Check sheet for the modelled part. Datum: model origin and axes. Units: mm. Face numbers are marked on the shaded views. A direction names the side the tool comes from. Coordinates: 2 decimals unless noted, no trailing zeros. Write each loop counter-clockwise with the first axis right and the second up, starting at its lowest first coordinate (ties: lowest second). Pieces come first, ordered by that corner, then holes. Notation, with made-up numbers: M 5.25,77.5 L 62.25,77.5 A21 ccw 62.25,86.5 Z; hole C 6.25,41.25 d6. An arc over 180 degrees is marked long. Answer as CSV lines item,"result". Start each with the question number.
Q1. Depth check by flat-ended pin: pin 1 Ø1.2 at (x, z) = (-8, -10) entering from +Y; pin 2 Ø1.5 at (x, y) = (-11.5, -3) entering from +Z; pin 3 Ø1.3 at (x, y) = (-26, -6.5) entering from -Z. Enter the tip coordinate at first touch or a pass-through.
Q2. Sectioned sample at D-D, the plane y = -2.5. Count the separate pieces of the cut face and the enclosed holes in it, then the cut area to 3 significant figures.
Q3. Sectioned sample at B-B, the plane x = 0. Record the cut outline in (y, z).
Q4. Sectioned sample at A-A, the plane z = 0. Record the cut outline in (x, y), then the cut area to 3 significant figures.
Q5. Mould release check, pull along X, two halves, no side actions. Record for the marked faces 3, 4 and 5: pulls with the +X half, pulls with the -X half, needs draft (parallel to the pull), parting line crosses it, or undercut.
Q6. Access from +Z, -Z, +X, -X, +Y, -Y to the whole of each face (thin tool, end or side, straight path). Record for the marked faces 1 and 2.
Q7. Thickness scan on line 1 along X through (y, z) = (-2, -26); line 2 along X through (y, z) = (-2.5, 26.25); line 3 along X through (y, z) = (-5.9, 0). Record the ranges inside material, lowest first. Write a range as from..to.
Q8. Sectioned sample at C-C, the plane z = -26.25. Record the cut outline in (x, y).
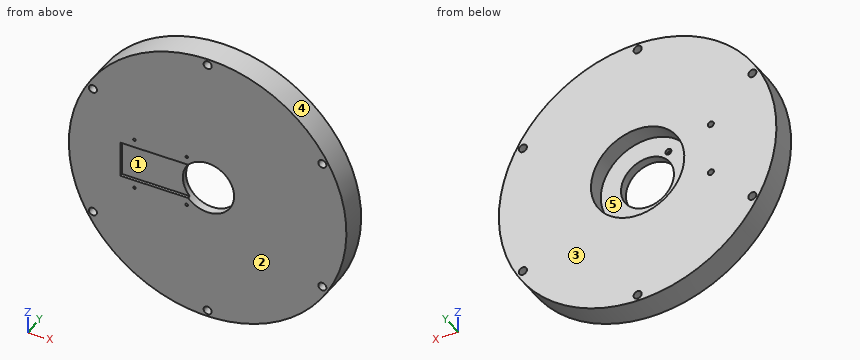
from build123d import *

# Parameters (mm, degrees)
SKETCH1_R           = 55
SKETCH1_R_2         = 50
SKETCH1_R_3         = 1.6
BOSS_EXTRUDE1_DEPTH = 7.5
SKETCH2_3_R         = 50
SKETCH2_3_R_2       = 10.5
BOSS_EXTRUDE2_DEPTH = 7.5
SKETCH2_R           = 0.5
CUT_EXTRUDE1_DEPTH  = 7.5
SKETCH2_3_2_R       = 1.2
SKETCH2_3_2_R_2     = 0.5
CUT_EXTRUDE2_DEPTH  = 5.3
CUT_EXTRUDE3_START  = -1.2
CUT_EXTRUDE3_DEPTH  = 1.2
SKETCH4_R           = 18.5
CUT_EXTRUDE4_DEPTH  = 4
BOSS_EXTRUDE3_START = 3
SKETCH5_R           = 55
SKETCH5_R_2         = 18.5
SKETCH5_R_3         = 1.6
SKETCH5_R_4         = 1.2
BOSS_EXTRUDE3_DEPTH = 3


with BuildPart() as part:
    # Sketch1 → Boss-Extrude1 (new body)
    with BuildSketch(Plane(origin=(0, 0, 0), x_dir=(1, 0, 0), z_dir=(0, 1, 0))):
        with Locations(Location((0, 0, 0), (0, 0, 270))):
            Circle(SKETCH1_R)
        with Locations(Location((0, 0, 0), (0, 0, 270))):
            Circle(SKETCH1_R_2, mode=Mode.SUBTRACT)
        with Locations(Location((0, 52.5, 0), (0, 0, 270))):
            Circle(SKETCH1_R_3, mode=Mode.SUBTRACT)
        with Locations(Location((45.466333699, 26.25, 0), (0, 0, 270))):
            Circle(SKETCH1_R_3, mode=Mode.SUBTRACT)
        with Locations(Location((45.466333699, -26.25, 0), (0, 0, 270))):
            Circle(SKETCH1_R_3, mode=Mode.SUBTRACT)
        with Locations(Location((0, -52.5, 0), (0, 0, 270))):
            Circle(SKETCH1_R_3, mode=Mode.SUBTRACT)
        with Locations(Location((-45.466333699, -26.25, 0), (0, 0, 270))):
            Circle(SKETCH1_R_3, mode=Mode.SUBTRACT)
        with Locations(Location((-45.466333699, 26.25, 0), (0, 0, 270))):
            Circle(SKETCH1_R_3, mode=Mode.SUBTRACT)
    extrude(amount=-BOSS_EXTRUDE1_DEPTH)

    # Sketch2_3 → Boss-Extrude2 (add)
    with BuildSketch(Plane(origin=(0, 0, 0), x_dir=(1, 0, 0), z_dir=(0, 1, 0))):
        Circle(SKETCH2_3_R)
        with Locations(Location((0, 0, 0), (0, 0, 270))):
            Circle(SKETCH2_3_R_2, mode=Mode.SUBTRACT)
    extrude(amount=-BOSS_EXTRUDE2_DEPTH)

    # Sketch2 → Cut-Extrude1 (cut)
    with BuildSketch(Plane(origin=(0, 0, 0), x_dir=(1, 0, 0), z_dir=(0, 1, 0))):
        with Locations(Location((-29, 10.25, 0), (0, 0, 270))):
            Circle(SKETCH2_R)
        with Locations(Location((-8.3, 10.25, 0), (0, 0, 270))):
            Circle(SKETCH2_R)
        with Locations(Location((-8.3, -10.25, 0), (0, 0, 270))):
            Circle(SKETCH2_R)
        with Locations(Location((-29, -10.25, 0), (0, 0, 270))):
            Circle(SKETCH2_R)
    extrude(amount=-CUT_EXTRUDE1_DEPTH, mode=Mode.SUBTRACT)

    # Sketch2_3 2 → Cut-Extrude2 (cut)
    # profile 1 of 4: a face of its own
    with BuildSketch(Plane(origin=(0, 0, 0), x_dir=(1, 0, 0), z_dir=(0, 1, 0))):
        with Locations(Location((-29, 10.25, 0), (0, 0, 270))):
            Circle(SKETCH2_3_2_R)
        with Locations(Location((-29, 10.25, 0), (0, 0, 270))):
            Circle(SKETCH2_3_2_R_2, mode=Mode.SUBTRACT)
    # profile 2 of 4: a face of its own
    with BuildSketch(Plane(origin=(0, 0, 0), x_dir=(1, 0, 0), z_dir=(0, 1, 0))):
        with Locations(Location((-8.3, 10.25, 0), (0, 0, 270))):
            Circle(SKETCH2_3_2_R)
        with Locations(Location((-8.3, 10.25, 0), (0, 0, 270))):
            Circle(SKETCH2_3_2_R_2, mode=Mode.SUBTRACT)
    # profile 3 of 4: a face of its own
    with BuildSketch(Plane(origin=(0, 0, 0), x_dir=(1, 0, 0), z_dir=(0, 1, 0))):
        with Locations(Location((-8.3, -10.25, 0), (0, 0, 270))):
            Circle(SKETCH2_3_2_R)
        with Locations(Location((-8.3, -10.25, 0), (0, 0, 270))):
            Circle(SKETCH2_3_2_R_2, mode=Mode.SUBTRACT)
    # profile 4 of 4: a face of its own
    with BuildSketch(Plane(origin=(0, 0, 0), x_dir=(1, 0, 0), z_dir=(0, 1, 0))):
        with Locations(Location((-29, -10.25, 0), (0, 0, 270))):
            Circle(SKETCH2_3_2_R)
        with Locations(Location((-29, -10.25, 0), (0, 0, 270))):
            Circle(SKETCH2_3_2_R_2, mode=Mode.SUBTRACT)
    extrude(amount=-CUT_EXTRUDE2_DEPTH, mode=Mode.SUBTRACT)

    # Sketch3 → Cut-Extrude3 (cut)
    with BuildSketch(Plane.XZ.offset(7.5).offset(CUT_EXTRUDE3_START)):
        with BuildLine():
            Line((-34.6, 0), (-10.5, 0))
            ThreePointArc((-10.5, 0), (-9.784532036, 3.809584338), (-7.735631842, 7.1))
            Line((-7.735631842, 7.1), (-34.6, 7.1))
            Line((-34.6, 7.1), (-34.6, 0))
        make_face()
        with BuildLine():
            ThreePointArc((-7.735631842, -7.1), (-9.784532036, -3.809584338), (-10.5, 0))
            Line((-10.5, 0), (-34.6, 0))
            Line((-34.6, 0), (-34.6, -7.1))
            Line((-34.6, -7.1), (-7.735631842, -7.1))
        make_face()
    extrude(amount=CUT_EXTRUDE3_DEPTH, mode=Mode.SUBTRACT)

    # Sketch4 → Cut-Extrude4 (cut)
    with BuildSketch(Plane(origin=(0, 0, 0), x_dir=(1, 0, 0), z_dir=(0, 1, 0))):
        with Locations(Location((0, 0, 0), (0, 0, 270))):
            Circle(SKETCH4_R)
    extrude(amount=-CUT_EXTRUDE4_DEPTH, mode=Mode.SUBTRACT)

    # Sketch5 → Boss-Extrude3 (add)
    with BuildSketch(Plane(origin=(0, 0, 0), x_dir=(1, 0, 0), z_dir=(0, 1, 0)).offset(BOSS_EXTRUDE3_START)):
        with Locations(Location((0, 0, 0), (0, 0, 270))):
            Circle(SKETCH5_R)
        with Locations(Location((0, 0, 0), (0, 0, 270))):
            Circle(SKETCH5_R_2, mode=Mode.SUBTRACT)
        with Locations(Location((0, 52.5, 0), (0, 0, 270))):
            Circle(SKETCH5_R_3, mode=Mode.SUBTRACT)
        with Locations(Location((-45.466333699, -26.25, 0), (0, 0, 270))):
            Circle(SKETCH5_R_3, mode=Mode.SUBTRACT)
        with Locations(Location((45.466333699, -26.25, 0), (0, 0, 270))):
            Circle(SKETCH5_R_3, mode=Mode.SUBTRACT)
        with Locations(Location((-29, -10.25, 0), (0, 0, 270))):
            Circle(SKETCH5_R_4, mode=Mode.SUBTRACT)
        with Locations(Location((45.466333699, 26.25, 0), (0, 0, 270))):
            Circle(SKETCH5_R_3, mode=Mode.SUBTRACT)
        with Locations(Location((0, -52.5, 0), (0, 0, 270))):
            Circle(SKETCH5_R_3, mode=Mode.SUBTRACT)
        with Locations(Location((-45.466333699, 26.25, 0), (0, 0, 270))):
            Circle(SKETCH5_R_3, mode=Mode.SUBTRACT)
        with Locations(Location((-29, 10.25, 0), (0, 0, 270))):
            Circle(SKETCH5_R_4, mode=Mode.SUBTRACT)
    extrude(amount=-BOSS_EXTRUDE3_DEPTH)


solid = part.part
Output:
1,pin 1,"stops at y = -5.3"
1,pin 2,"stops at z = 53.94"
1,pin 3,"stops at z = -48.81"
2,separate pieces,"1"
2,enclosed holes,"9"
2,area,"8,370 mm^2"
3,outline,"M -7.5,-55 L 3,-55 L 3,-54.1 L -7.5,-54.1 Z; M -7.5,-50.9 L 3,-50.9 L 3,-18.5 L -4,-18.5 L -4,-10.5 L -7.5,-10.5 Z; M -7.5,10.5 L -4,10.5 L -4,18.5 L 3,18.5 L 3,50.9 L -7.5,50.9 Z; M -7.5,54.1 L 3,54.1 L 3,55 L -7.5,55 Z"
4,outline,"M -55,-7.5 L -34.6,-7.5 L -34.6,-6.3 L -10.5,-6.3 L -10.5,-4 L -18.5,-4 L -18.5,3 L -55,3 Z; M 10.5,-7.5 L 55,-7.5 L 55,3 L 18.5,3 L 18.5,-4 L 10.5,-4 Z"
4,area,"794 mm^2"
5,face 3,"needs draft"
5,face 4,"parting line crosses it"
5,face 5,"undercut"
6,face 1,"-Y"
6,face 2,"+Z, -Z, +X, -X, -Y"
7,line 1,"x = -48.47..-47.05, -43.89..43.89, 47.05..48.47"
7,line 2,"x = -48.33..-47.07, -43.87..43.87, 47.07..48.33"
7,line 3,"x = -55..-10.5, 10.5..55"
8,outline,"M -48.33,-7.5 L -47.07,-7.5 L -47.07,3 L -48.33,3 Z; M -43.87,-7.5 L 43.87,-7.5 L 43.87,3 L -43.87,3 Z; M 47.07,-7.5 L 48.33,-7.5 L 48.33,3 L 47.07,3 Z"
